Here's the drawing with two shaded views (mm, measured from the low corner). I have some questions. Round coordinates to 2 decimals unless told otherwise and drop trailing zeros. Loops run counter-clockwise (first coordinate to the right, second up) from the corner with the lowest first, then second, coordinate; pieces in that order, holes last. Notation, with made-up numbers: (16.25, 69.5) -> (56.25, 69.5) arc R22 ccw to (56.25, 77.5) -> close; hole circle Ø3 at (-11.5, 77). An arc over 180 degrees is marked (long way). Use a Markdown table: item, result.
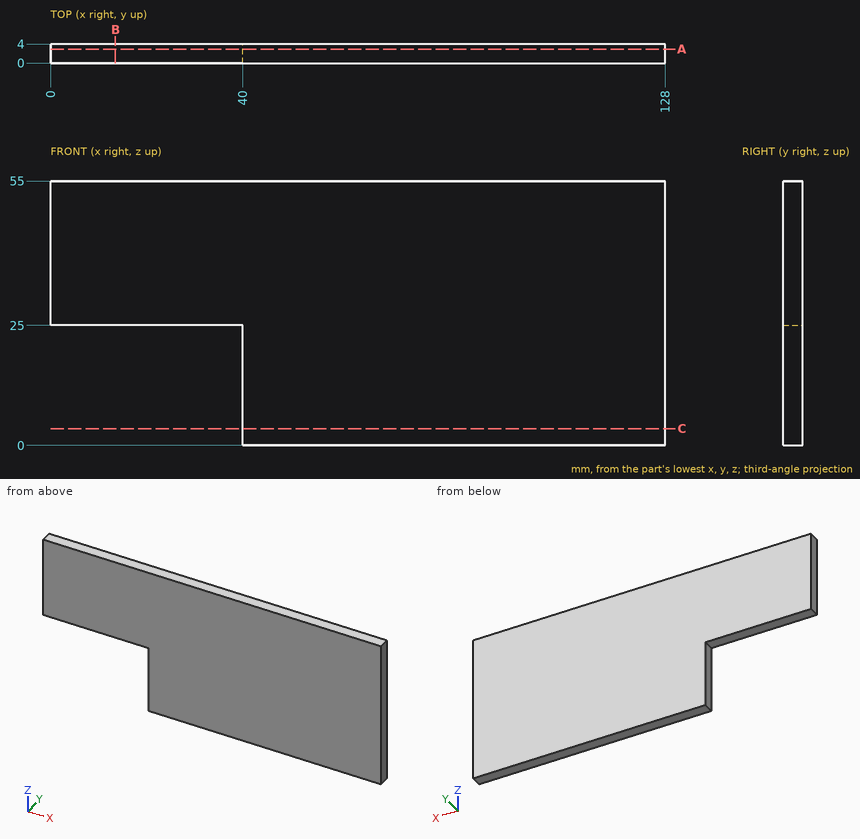
1. I want a section at C-C (z = 3.5). Please give me the cut outline in (x, y).
Answer sheet:
| item | result |
|---|---|
| outline | (40, 0) -> (128, 0) -> (128, 4) -> (40, 4) -> close |
2. I want a section at B-B (x = 13.5). Please give me the cut outline in (y, z).
Answer sheet:
| item | result |
|---|---|
| outline | (0, 25) -> (4, 25) -> (4, 55) -> (0, 55) -> close |
3. I want a section at A-A (y = 2.95). Please give me the cut outline in (x, z).
Answer sheet:
| item | result |
|---|---|
| outline | (0, 25) -> (40, 25) -> (40, 0) -> (128, 0) -> (128, 55) -> (0, 55) -> close |
4. I need wall thicknesses on line 1 (Z direction, x = 8, y = 1.3); line 2 (X direction, y = 1.7, z = 11). Which ranges of each line are inside material? Lowest first, please.
Answer sheet:
| item | result |
|---|---|
| line 1 | z = 25 to 55 |
| line 2 | x = 40 to 128 |
